Here's how the part is built. I have some questions about the finished solid (model axes, mm). Face numbers are marked on the shaded views. A direction names the side the tool comes from. Give positions to 0.01 mm unless a question says otherwise; leave off trailing zeros. Loops run counter-clockwise (first coordinate to the right, second up) from the corner with the lowest first, then second, coordinate; pieces in that order, holes last. Notation, with made-up numbers: (73.25, -14.75) -> (88.25, -14.75) arc R13 cw to (88.25, -3.75) -> close; hole circle Ø8 at (43, 65). An arc over 180 degrees is marked (long way). Answer in a Markdown table with one row per item. Add a question column.
Item 1: If I drill on line 1 (X direction, y = -14, z = 11); line 2 (Y direction, x = 0, z = 74); line 3 (Z direction, x = 23.5, y = -9), over which ranges is the centre line in solid material (lowest first)?
Item 2: For P1, Ø7.5, axis at x = -3, y = 31, coming from the +Z side; P2, Ø1.5, axis at x = -15, z = 9, coming from the +Y side; P3, Ø11, axis at x = 24.5, y = -12.5, coming from the +Z side; P4, Ø10.5, axis at x = 1.5, y = -0.5, coming from the +Z side, each with a flat end and sliding along its axis, tell me the tip position at first contact or that it passes through.
Item 3: We'd pull the mould along Z, two halves only. Please class the marked faces 4, 5 and 6: released by +Z, released by -Z, zero draft, split by the parting line, or undercut.
Item 4: If we section it at C-C (z = 22): Write out the boundary of the cut face in (x, y), then the cut area to 3 significant figures.
Item 5: If we section it at D-D (z = 67): Write out the boundary of the cut face in (x, y).
Item 6: If we section it at A-A (x = -28): Write out the boundary of the cut face in (y, z), then the cut area to 3 significant figures.
Item 7: If we section it at B-B (y = 29): Write out the boundary of the cut face in (x, z), then the cut area to 3 significant figures.
Item 8: Which directions (+Z, -Z, +X, -X, +Y, -Y) give clear straight access to the entire face, cutting with the end or side of a thin tool? Please do the marked faces 1, 2 and 3.
```python
from build123d import *

# Parameters (mm, degrees)
SKETCH1_R           = 4
BOSS_EXTRUDE1_DEPTH = 20
SKETCH2_R           = 15
BOSS_EXTRUDE2_DEPTH = 9
SKETCH3_R           = 12.5
BOSS_EXTRUDE3_DEPTH = 45
SKETCH5_R           = 15
BOSS_EXTRUDE4_DEPTH = 10
FILLET3_R           = 9
FILLET4_R           = 15
SKETCH6_R           = 4.75
CUT_EXTRUDE1_DEPTH  = 20


with BuildPart() as part:
    # Sketch1 → Boss-Extrude1 (new body)
    with BuildSketch(Plane.XY):
        with BuildLine():
            Line((10.311065776, 31.812768666), (13.037811649, 7.527384065))
            Line((13.037811649, 7.527384065), (32.706198717, -6.976739431))
            ThreePointArc((32.706198717, -6.976739431), (34.146892061, -8.992770752), (34.123690383, -11.470560347))
            ThreePointArc((34.123690383, -11.470560347), (31.176914536, -18), (26.995641847, -23.816702569))
            ThreePointArc((26.995641847, -23.816702569), (24.861413952, -25.075690609), (22.395132941, -24.836029235))
            Line((22.395132941, -24.836029235), (0, -15.05476813))
            Line((0, -15.05476813), (-22.395132941, -24.836029235))
            ThreePointArc((-22.395132941, -24.836029235), (-24.861413952, -25.075690609), (-26.995641847, -23.816702569))
            ThreePointArc((-26.995641847, -23.816702569), (-31.176914536, -18), (-34.123690383, -11.470560347))
            ThreePointArc((-34.123690383, -11.470560347), (-34.146892061, -8.992770752), (-32.706198717, -6.976739431))
            Line((-32.706198717, -6.976739431), (-13.037811649, 7.527384065))
            Line((-13.037811649, 7.527384065), (-10.311065776, 31.812768666))
            ThreePointArc((-10.311065776, 31.812768666), (-9.285478109, 34.068461361), (-7.128048535, 35.287262916))
            ThreePointArc((-7.128048535, 35.287262916), (0, 36), (7.128048535, 35.287262916))
            ThreePointArc((7.128048535, 35.287262916), (9.285478109, 34.068461361), (10.311065776, 31.812768666))
        make_face()
        with Locations((0, 29)):
            Circle(SKETCH1_R, mode=Mode.SUBTRACT)
        with Locations((-25.11473671, -14.5)):
            Circle(SKETCH1_R, mode=Mode.SUBTRACT)
        with Locations((25.11473671, -14.5)):
            Circle(SKETCH1_R, mode=Mode.SUBTRACT)
    extrude(amount=BOSS_EXTRUDE1_DEPTH)

    # Sketch2 → Boss-Extrude2 (add)
    with BuildSketch(Plane.XY.offset(20)):
        with Locations(Location((0, 0, 0), (0, 0, 180))):
            Circle(SKETCH2_R)
    extrude(amount=BOSS_EXTRUDE2_DEPTH)

    # Sketch3 → Boss-Extrude3 (add)
    with BuildSketch(Plane.XY.offset(29)):
        with Locations(Location((0, 0, 0), (0, 0, 180))):
            Circle(SKETCH3_R)
    extrude(amount=BOSS_EXTRUDE3_DEPTH)

    # Sketch5 → Boss-Extrude4 (add)
    with BuildSketch(Plane.XY.offset(74)):
        with Locations(Location((0, 0, 0), (0, 0, 180))):
            Circle(SKETCH5_R)
    extrude(amount=BOSS_EXTRUDE4_DEPTH)

    # Fillet3
    # the kernel refuses this fillet: 9 mm, written as the material it adds along each edge
    with BuildSketch(Plane(origin=(0, 0, 20), x_dir=(-1, 0, 0), z_dir=(0, 1, 0))) as fillet3_piece_1_section:
        with BuildLine():
            CenterArc((15 + FILLET3_R, FILLET3_R), FILLET3_R, 180, 90)
            Line((15 + FILLET3_R, 0), (15, 0))
            Line((15, 0), (15, FILLET3_R))
        make_face()
    fillet3_piece_1 = revolve(axis=Axis((0, 0, 20), (0, 0, 1)), mode=Mode.PRIVATE)
    fillet3_piece_1 = split(fillet3_piece_1, bisect_by=Plane(origin=(-2.104235359, 18.693633693, 22.074494406), z_dir=(-0.5935073720778344, -0.8048285527298736, 0)), keep=Keep.TOP, mode=Mode.PRIVATE)
    fillet3_piece_1 = split(fillet3_piece_1, bisect_by=Plane(origin=(-19.127560762, 3.036600307, 22.074494406), z_dir=(0.5935073720778299, -0.8048285527298771, 0)), keep=Keep.TOP, mode=Mode.PRIVATE)
    fillet3_piece_1 = split(fillet3_piece_1, bisect_by=Plane(origin=(-8.489861011, -18.762785739, 22.074494406), z_dir=(-0.4002482863162174, 0.9164067379176843, 0)), keep=Keep.TOP, mode=Mode.PRIVATE)
    add(fillet3_piece_1)
    with BuildSketch(Plane(origin=(0, 0, 20), x_dir=(-1, 0, 0), z_dir=(0, 1, 0))) as fillet3_piece_2_section:
        with BuildLine():
            CenterArc((15 + FILLET3_R, FILLET3_R), FILLET3_R, 180, 90)
            Line((15 + FILLET3_R, 0), (15, 0))
            Line((15, 0), (15, FILLET3_R))
        make_face()
    fillet3_piece_2 = revolve(axis=Axis((0, 0, 20), (0, 0, 1)), mode=Mode.PRIVATE)
    fillet3_piece_2 = split(fillet3_piece_2, bisect_by=Plane(origin=(12.004118745, 16.733826801, 22.074494266), z_dir=(-0.9937556583940517, -0.11157818518780918, 0)), keep=Keep.TOP, mode=Mode.PRIVATE)
    fillet3_piece_2 = split(fillet3_piece_2, bisect_by=Plane(origin=(-12.193553488, 15.046652486, 22.074494266), z_dir=(0.9937556583940516, -0.1115781851878097, 0)), keep=Keep.TOP, mode=Mode.PRIVATE)
    fillet3_piece_2 = split(fillet3_piece_2, bisect_by=Plane(origin=(-17.241277087, -7.524496557, 22.074494266), z_dir=(0.4002482863162113, 0.916406737917687, 0)), keep=Keep.TOP, mode=Mode.PRIVATE)
    add(fillet3_piece_2)
    with BuildSketch(Plane(origin=(0, 0, 20), x_dir=(-1, 0, 0), z_dir=(0, 1, 0))) as fillet3_piece_3_section:
        with BuildLine():
            CenterArc((15 + FILLET3_R, FILLET3_R), FILLET3_R, 180, 90)
            Line((15 + FILLET3_R, 0), (15, 0))
            Line((15, 0), (15, FILLET3_R))
        make_face()
    fillet3_piece_3 = revolve(axis=Axis((0, 0, 20), (0, 0, 1)), mode=Mode.PRIVATE)
    fillet3_piece_3 = split(fillet3_piece_3, bisect_by=Plane(origin=(12.39704086, -20.469279127, 20.602322319), z_dir=(0.4002482863162113, 0.916406737917687, 0)), keep=Keep.TOP, mode=Mode.PRIVATE)
    fillet3_piece_3 = split(fillet3_piece_3, bisect_by=Plane(origin=(16.223816266, -7.968881057, 20.602322319), z_dir=(0.4002482863162174, -0.9164067379176843, 0)), keep=Keep.TOP, mode=Mode.PRIVATE)
    add(fillet3_piece_3)

    # Fillet4
    # the kernel refuses this fillet: 15 mm, written as the material it adds along each edge
    with BuildSketch(Plane(origin=(0, 0, 29), x_dir=(-1, 0, 0), z_dir=(0, 1, 0))) as fillet4_piece_1:
        with BuildLine():
            CenterArc((27.5, 8.291561976), FILLET4_R, 180, 33.557309762)
            Line((12.5, 8.291561976), (12.5, 0))
            Line((12.5, 0), (15, 0))
        make_face()
    revolve(axis=Axis((0, 0, 29), (0, 0, 1)))
    with BuildSketch(Plane(origin=(0, 0, 74), x_dir=(-1, 0, 0), z_dir=(0, 1, 0))) as fillet4_piece_2:
        with BuildLine():
            CenterArc((27.5, -8.291561976), FILLET4_R, 146.442690238, 33.557309762)
            Line((15, 0), (12.5, 0))
            Line((12.5, 0), (12.5, -8.291561976))
        make_face()
    revolve(axis=Axis((0, 0, 74), (0, 0, 1)))

    # Sketch6 → Cut-Extrude1 (cut)
    with BuildSketch(Plane.XY.offset(84)):
        Circle(SKETCH6_R)
    extrude(amount=-CUT_EXTRUDE1_DEPTH, mode=Mode.SUBTRACT)


solid = part.part
```
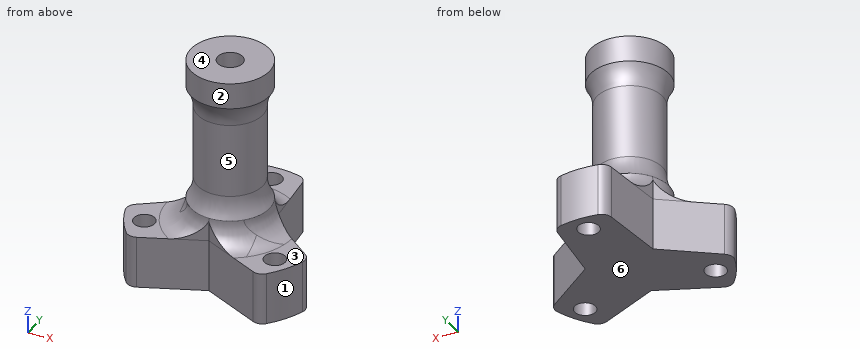
Recorded:
| question | item | result |
|---|---|---|
| 1 | line 1 | x = -33.17 to -29.08, -21.15 to 21.15, 29.08 to 33.17 |
| 1 | line 2 | y = -15 to -4.75, 4.75 to 15 |
| 1 | line 3 | z = 0 to 20 |
| 2 | P1 | stops at z = 20 |
| 2 | P2 | stops at y = 6.63 |
| 2 | P3 | stops at z = 20.22 |
| 2 | P4 | stops at z = 84 |
| 3 | face 4 | released by +Z |
| 3 | face 5 | undercut |
| 3 | face 6 | released by -Z |
| 4 | outline | (-17.92, 3.93) arc R18.34 ccw to (-5.56, -17.48) -> (0, -15.05) -> (5.56, -17.48) arc R18.34 ccw to (17.92, 3.93) -> (13.04, 7.53) -> (12.36, 13.55) arc R18.34 ccw to (-12.36, 13.55) -> (-13.04, 7.53) -> close |
| 4 | area | 997 mm^2 |
| 5 | outline | circle Ø25.11 at (0, 0); hole circle Ø9.5 at (0, 0) |
| 6 | outline | (-22.63, 0) -> (-17.27, 0) -> (-17.27, 20) -> (-22.63, 20) -> close; (-11.73, 0) -> (-3.51, 0) -> (-3.51, 20) -> (-11.73, 20) -> close |
| 6 | area | 272 mm^2 |
| 7 | outline | (-10.63, 0) -> (-4, 0) -> (-4, 20) -> (-10.63, 20) -> close; (4, 0) -> (10.63, 0) -> (10.63, 20) -> (4, 20) -> close |
| 7 | area | 265 mm^2 |
| 8 | face 1 | +Z, -Z, +X, -Y |
| 8 | face 2 | +Z |
| 8 | face 3 | +Z, +X, -Y |
